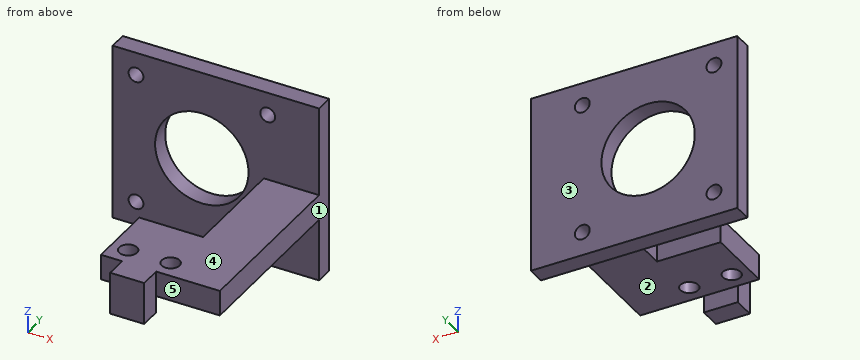
from build123d import *

# Parameters (mm, degrees)
SKETCH_1_W          = 18
SKETCH_1_H          = 50
EXTRUDE_1_DEPTH     = 6
SKETCH_3_R          = 2.1
CUT_EXTRUDE_2_DEPTH = 6
SKETCH_4_W          = 8
SKETCH_4_H          = 10
EXTRUDE_2_DEPTH     = 5
SKETCH_5_W          = 6
SKETCH_5_H          = 50
EXTRUDE_3_DEPTH     = 10
SKETCH_6_W          = 15
SKETCH_6_H          = 33.880633875
CUT_EXTRUDE_3_DEPTH = 10
SKETCH_7_W          = 18.194641251
SKETCH_7_H          = 8.438338953
CUT_EXTRUDE_4_DEPTH = 4.2
SKETCH_8_W          = 58.547266504
SKETCH_8_H          = 42
EXTRUDE_4_DEPTH     = 4.2
SKETCH_9_W          = 49.225807408
SKETCH_9_H          = 6.051517764
CUT_EXTRUDE_5_DEPTH = 9.95
SKETCH_15_R         = 1.75
CUT_EXTRUDE_6_DEPTH = 9.95
SKETCH_16_R         = 11
CUT_EXTRUDE_7_DEPTH = 10


with BuildPart() as part:
    # 草图1 → 凸台-拉伸1 (new body)
    with BuildSketch(Plane.XY):
        with Locations((9, 25)):
            Rectangle(SKETCH_1_W, SKETCH_1_H)
    extrude(amount=EXTRUDE_1_DEPTH)

    # 草图3 → 切除-拉伸2 (cut)
    with BuildSketch(Plane.XY.offset(6)):
        with Locations((4, 4.30447472)):
            Circle(SKETCH_3_R)
        with Locations((14, 4.30447472)):
            Circle(SKETCH_3_R)
    extrude(amount=-CUT_EXTRUDE_2_DEPTH, mode=Mode.SUBTRACT)

    # 草图4 → 凸台-拉伸2 (add)
    with BuildSketch(Plane.XZ):
        with Locations((9, 1)):
            Rectangle(SKETCH_4_W, SKETCH_4_H)
    extrude(amount=EXTRUDE_2_DEPTH)

    # 草图5 → 凸台-拉伸3 (add)
    with BuildSketch(Plane(origin=(18, 0, 0), x_dir=(0, 0, -1), z_dir=(1, 0, 0))):
        with Locations((-3, 25)):
            Rectangle(SKETCH_5_W, SKETCH_5_H)
    extrude(amount=EXTRUDE_3_DEPTH)

    # 草图6 → 切除-拉伸3 (cut)
    with BuildSketch(Plane.XY.offset(6)):
        with Locations((7.5, 33.059683062)):
            Rectangle(SKETCH_6_W, SKETCH_6_H)
    extrude(amount=-CUT_EXTRUDE_3_DEPTH, mode=Mode.SUBTRACT)

    # 草图7 → 切除-拉伸4 (cut)
    with BuildSketch(Plane(origin=(0, 50, 0), x_dir=(1, 0, 0), z_dir=(0, 1, 0))):
        with Locations((18.902679374, -1.780830523)):
            Rectangle(SKETCH_7_W, SKETCH_7_H)
    extrude(amount=-CUT_EXTRUDE_4_DEPTH, mode=Mode.SUBTRACT)

    # 草图8 → 凸台-拉伸4 (add)
    with BuildSketch(Plane(origin=(0, 45.8, 0), x_dir=(1, 0, 0), z_dir=(0, 1, 0))):
        with Locations((-1.273633252, -6.17)):
            Rectangle(SKETCH_8_W, SKETCH_8_H)
    extrude(amount=-EXTRUDE_4_DEPTH)

    # 草图9 → 切除-拉伸5 (cut)
    with BuildSketch(Plane.ZY.offset(30.547266504)):
        with Locations((2.557096296, 42.774241118)):
            Rectangle(SKETCH_9_W, SKETCH_9_H)
    extrude(amount=-CUT_EXTRUDE_5_DEPTH, mode=Mode.SUBTRACT)

    # 草图15 → 切除-拉伸6 (cut)
    with BuildSketch(Plane.XZ.offset(-41.6)):
        with Locations((15.90237217, -9.22379542)):
            Circle(SKETCH_15_R)
        with Locations((-15.09762783, -9.22379542)):
            Circle(SKETCH_15_R)
        with Locations((15.90237217, 21.77620458)):
            Circle(SKETCH_15_R)
        with Locations((-15.09762783, 21.77620458)):
            Circle(SKETCH_15_R)
    extrude(amount=-CUT_EXTRUDE_6_DEPTH, mode=Mode.SUBTRACT)

    # 草图16 → 切除-拉伸7 (cut)
    with BuildSketch(Plane.XZ.offset(-41.6)):
        with Locations((0.40237217, 6.27620458)):
            Circle(SKETCH_16_R)
    extrude(amount=-CUT_EXTRUDE_7_DEPTH, mode=Mode.SUBTRACT)


solid = part.part
Geometry check sheet. Reference: the model listing, model coordinates, mm. Face numbers are marked on the shaded views. A direction names the side the tool comes from. Give positions to 0.01 mm unless a question says otherwise; leave off trailing zeros. Order: outer loops, then holes, each group sorted by start corner. A loop starts at its lowest first (then second) coordinate and runs counter-clockwise, first axis right, second up.
1. Access from +Z, -Z, +X, -X, +Y, -Y to the whole of each face (thin tool, end or side, straight path). Record for the marked faces 1, 2, 3, 4 and 5.
Completed:
face 1: +Z, -Z, +X, +Y, -Y
face 2: -Z, +X, -X
face 3: +Z, -Z, +X, -X, +Y
face 4: +Z, +X, -X, -Y
face 5: +Z, -Z, +X, -Y
2. Scan lines: line 1 (Y direction, x = 14, z = 3.45); line 2 (Y direction, x = 4, z = 2); line 3 (X direction, y = 35, z = 5). Record each from-to range of solid material in increasing order.
Completed:
line 1: y = 0 to 2.2, 6.4 to 16.12, 41.6 to 45.8
line 2: y = 0 to 2.2, 6.4 to 16.12
line 3: x = 15 to 28
3. Sectioned sample at D-D (y = 9.5). Record the boundary of the cut face in (x, z).
Completed:
outline: (0, 0) - (28, 0) - (28, 6) - (0, 6) - close
4. Sectioned sample at C-C (x = 4). Record the boundary of the cut face in (y, z).
Completed:
outline: (0, 0) - (2.2, 0) - (2.2, 6) - (0, 6) - close; (6.4, 0) - (16.12, 0) - (16.12, 6) - (6.4, 6) - close; (41.6, -14.83) - (45.8, -14.83) - (45.8, -4.12) - (41.6, -4.12) - close; (41.6, 16.67) - (45.8, 16.67) - (45.8, 27.17) - (41.6, 27.17) - close
5. Depth check by flat-ended pin: pin 1 (1.8 mm diameter, centred on y = 11, z = 4, fed in from -X); pin 2 (6.5 mm diameter, centred on x = 14, y = 4.3, fed in from -Z); pin 3 (6.5 mm diameter, centred on x = 22, z = 4, fed in from -Y); pin 4 (12.5 mm diameter, centred on x = 14.5, z = 11, fed in from -Y). Enter the tip coordinate at first touch or a pass-through.
Completed:
pin 1: stops at x = 0
pin 2: stops at z = 0
pin 3: stops at y = 0
pin 4: stops at y = -5
6. Sectioned sample at A-A (x = 24.5). Record the boundary of the cut face in (y, z).
Completed:
outline: (0, 0) - (41.6, 0) - (41.6, -14.83) - (45.8, -14.83) - (45.8, 27.17) - (41.6, 27.17) - (41.6, 6) - (0, 6) - close
7. Sectioned sample at B-B (z = -1). Record the boundary of the cut face in (x, y), then the cut area to 3 significant figures.
Completed:
outline: (-20.6, 41.6) - (-7.85, 41.6) - (-7.85, 45.8) - (-20.6, 45.8) - close; (5, -5) - (13, -5) - (13, 0) - (5, 0) - close; (8.65, 41.6) - (28, 41.6) - (28, 45.8) - (8.65, 45.8) - close
area: 175 mm2
